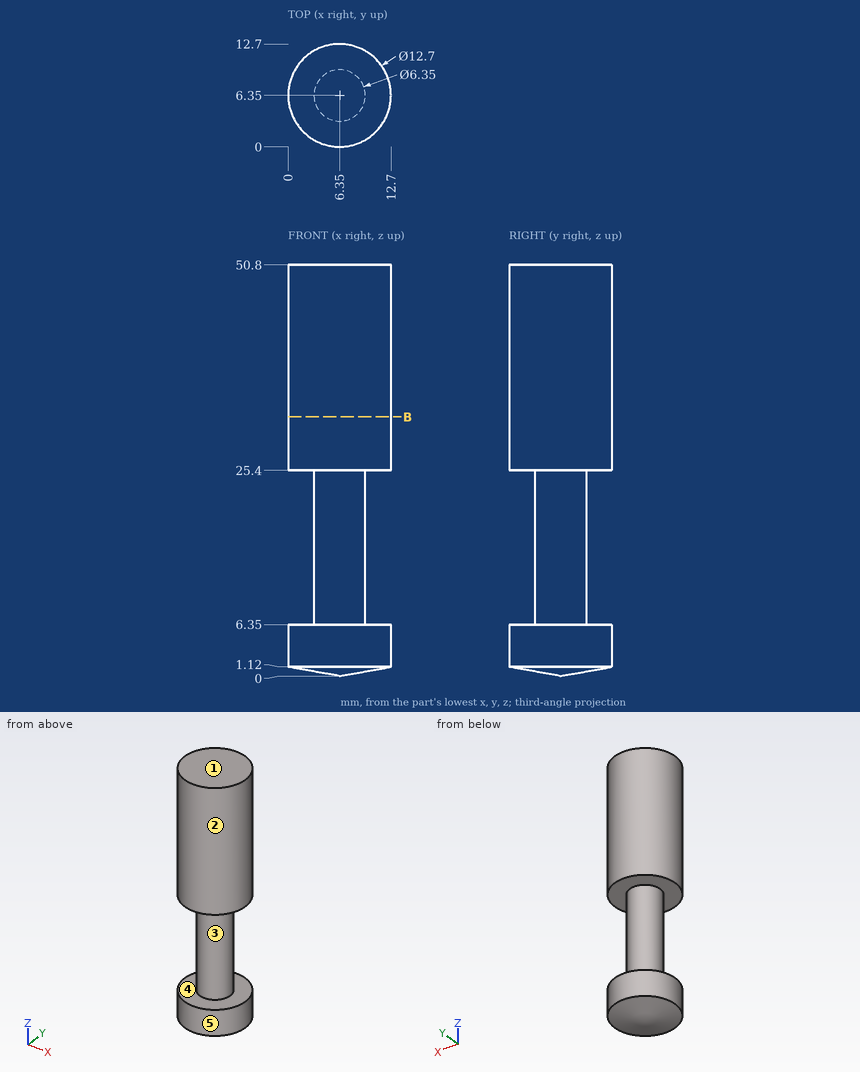
The figure shows three views and two pictorial views of one solid part (mm, origin at its lowest corner). Answer the questions. A direction names the side the tool comes from. Round coordinates to 2 decimals unless told otherwise and drop trailing zeros. Order: outer loops, then holes, each group sorted by start corner. A loop starts at its lowest first (then second) coordinate and runs counter-clockwise, first axis right, second up. Notation, with made-up numbers: M 89,2.5 L 97,2.5 A27 ccw 97,22.5 Z; hole C 20.5,-12 d3. An arc over 180 degrees is marked long. Answer in a Markdown table with one row per item. Add a question column.
1) Which of the six approach directions +Z, -Z, +X, -X, +Y, -Y give full straight-line access (tool end or side, diameter ignored) to the marked faces 4 and 5?
2) Determine the mould class of the marked faces 1, 2 and 3 for opening direction Z: pulls with the +Z half, pulls with the -Z half, needs draft (parallel to the pull), parting line crosses it, or undercut.
3) Flat-ended cylindrical pins translate along their axes: pin 1 Ø1.5 at (x, z) = (9, 12.5) entering from +Y; pin 2 Ø3 at (y, z) = (9, 20.5) entering from +X; pin 3 Ø2 at (y, z) = (9, 25) entering from +X. Find the tip coordinate at first contact, or state that the pin passes through.
4) Consider line 1 along Z through (x, y) = (3.75, 2.5); line 2 along Z through (x, y) = (6, 0.5); line 3 along X through (y, z) = (6.5, 9). Determine where each line is inside the solid, lowest interval first. Write a range as from..to.
5) The part is cut by section B-B on z = 32. Determine the outline of the cut face in (x, y).
Findings below:
| question | item | result |
|---|---|---|
| 1 | face 4 | none |
| 1 | face 5 | +Z, -Z |
| 2 | face 1 | pulls with the +Z half |
| 2 | face 2 | needs draft |
| 2 | face 3 | undercut |
| 3 | pin 1 | stops at y = 8.89 |
| 3 | pin 2 | stops at x = 9.31 |
| 3 | pin 3 | stops at x = 12.46 |
| 4 | line 1 | z = 0.82..6.35, 25.4..50.8 |
| 4 | line 2 | z = 1.03..6.35, 25.4..50.8 |
| 4 | line 3 | x = 3.18..9.52 |
| 5 | outline | C 6.35,6.35 d12.7 |
